```python
from build123d import *

# Parameters (mm, degrees)
F1_DEPTH = 25.4
F2_W     = 78.052774
F2_H     = 28.209937
F3_DEPTH = 12.7


with BuildPart() as f1:
    # F0 (on Front) → F1 (new body)
    with BuildSketch(Plane.XZ):
        with BuildLine():
            Line((51.145062, 20.566268), (-33.970713, 20.566268))
            ThreePointArc((-33.970713, 20.566268), (-38.460841, 18.706396), (-40.320713, 14.216268))
            Line((-40.320713, 14.216268), (-40.320713, -20.385863))
            Line((-40.320713, -20.385863), (51.145062, -20.385863))
            Line((51.145062, -20.385863), (51.145062, 20.566268))
        make_face()
    extrude(amount=F1_DEPTH)

    # F2 (on face) → F3 (cut)
    with BuildSketch(Plane.XZ.offset(25.4)):
        with Locations((6.687261, -0.101787)):
            Rectangle(F2_W, F2_H)
    extrude(amount=-F3_DEPTH, mode=Mode.SUBTRACT)


solid = f1.part
```
Source: CAD feature listing. Evaluate the final solid. Frame: model axes, mm. A direction names the side the tool comes from. Give positions to 0.01 mm unless a question says otherwise; leave off trailing zeros. Loops run counter-clockwise (first coordinate to the right, second up) from the corner with the lowest first, then second, coordinate; pieces in that order, holes last. Notation, with made-up numbers: (-25.75, -21) -> (27.25, -21) arc R22 ccw to (27.25, -9) -> close; hole circle Ø2 at (21.25, 58). An arc over 180 degrees is marked (long way). Put each result on its own line as item: value. Start each with the question number.
1) Cut plane C-C (z = 3.5). Return loops of the section in (x, y), then the cut area to 3 significant figures.
2) Cut plane B-B (x = -9.5). Return loops of the section in (y, z).
3) Cut plane A-A (y = -17.5). Return loops of the section in (x, z), then the cut area to 3 significant figures.
4) Reachability of faces 5 (the face through (45.714, -19, 0)), 6 (the face through (9, -13, 20.566)) from +Z, -Z, +X, -X, +Y, -Y: full face, straight path, thin tool, end or side. Return the list, or none.
5) Material intervals for probe 1 along Z at (x, y) = (-0.5, -15.25); probe 2 along X at (y, z) = (-20.25, 13.5); probe 3 along Y at (x, z) = (-7, -0.5), sorted ascending.
6) Draft query along X for faces 1 (the face through (6, -19, 14.003)), 2 (the face through (5, 0, 0)), 3 (the face through (-38.411, -12.522, 18.755)), 4 (the face through (6, -12.7, 0)). Return one class per face: released by +X, released by -X, zero draft, split by the parting line, or undercut.
7) Contact query for a flat-ended pin moving along its axis: P1, Ø1, axis at x = 8.5, z = -3.5, coming from the -Y side. Output: stop coordinate, or through.
Results are:
1. outline: (-40.32, -25.4) -> (-32.34, -25.4) -> (-32.34, -12.7) -> (45.71, -12.7) -> (45.71, -25.4) -> (51.15, -25.4) -> (51.15, 0) -> (-40.32, 0) -> close
1. area: 1,330 mm2
2. outline: (-25.4, -20.39) -> (0, -20.39) -> (0, 20.57) -> (-25.4, 20.57) -> (-25.4, 14) -> (-12.7, 14) -> (-12.7, -14.21) -> (-25.4, -14.21) -> close
3. outline: (-40.32, -20.39) -> (51.15, -20.39) -> (51.15, 20.57) -> (-33.97, 20.57) arc R6.35 ccw to (-40.32, 14.22) -> close; hole (-32.34, -14.21) -> (45.71, -14.21) -> (45.71, 14) -> (-32.34, 14) -> close
3. area: 1,540 mm2
4. face 5: -Y
4. face 6: +Z, +X, -X, +Y, -Y
5. probe 1: z = -20.39 to -14.21, 14 to 20.57
5. probe 2: x = -40.32 to -32.34, 45.71 to 51.15
5. probe 3: y = -12.7 to 0
6. face 1: undercut
6. face 2: zero draft
6. face 3: released by -X
6. face 4: undercut
7. P1: stops at y = -12.7
